For this review, take the finished solid that the model builds, in its own axes (mm). Coordinates: 2 decimals unless noted, no trailing zeros. Loops run counter-clockwise (first coordinate to the right, second up) from the corner with the lowest first, then second, coordinate; pieces in that order, holes last. Notation, with made-up numbers: (-10.5, 76) -> (38.5, 76) arc R28 cw to (38.5, 114) -> close; hole circle Ø9 at (-27.75, 15). An arc over 180 degrees is marked (long way). Use a Markdown table: item, result.
from build123d import *

# Parameters (mm, degrees)
CROQUIS1_W              = 580
CROQUIS1_H              = 80
CROQUIS1_R              = 12.6
SALIENTE_EXTRUIR1_DEPTH = 16


with BuildPart() as part:
    # Croquis1 → Saliente-Extruir1 (new body)
    with BuildSketch(Plane.XY):
        Rectangle(CROQUIS1_W, CROQUIS1_H)
        with Locations((-240, -20)):
            Circle(CROQUIS1_R, mode=Mode.SUBTRACT)
        with Locations((-120, -20)):
            Circle(CROQUIS1_R, mode=Mode.SUBTRACT)
        with Locations((0, -20)):
            Circle(CROQUIS1_R, mode=Mode.SUBTRACT)
        with Locations((120, -20)):
            Circle(CROQUIS1_R, mode=Mode.SUBTRACT)
        with Locations((240, -20)):
            Circle(CROQUIS1_R, mode=Mode.SUBTRACT)
    extrude(amount=-SALIENTE_EXTRUIR1_DEPTH)


solid = part.part
(1) Mouldability with a two-part tool opening along Y and no side actions: class faces 1 (the face through (-4, 40, -8)), 2 (the face through (227.412, -19.446, -7.888)), 3 (the face through (-4, 1, 0)) as pulls with the +Y half, pulls with the -Y half, needs draft (parallel to the pull), parting line crosses it, or undercut.
Found:
| item | result |
|---|---|
| face 1 | pulls with the +Y half |
| face 2 | undercut |
| face 3 | needs draft |
(2) For line 1 along X through (y, z) = (-18.5, -10.5); line 2 along Y through (x, z) = (-120, -6.75); line 3 along X through (y, z) = (-25.5, -10.75), list the stretches that pass through material, from the lowest coordinate up.
Found:
| item | result |
|---|---|
| line 1 | x = -290 to -252.51, -227.49 to -132.51, -107.49 to -12.51, 12.51 to 107.49, 132.51 to 227.49, 252.51 to 290 |
| line 2 | y = -40 to -32.6, -7.4 to 40 |
| line 3 | x = -290 to -251.34, -228.66 to -131.34, -108.66 to -11.34, 11.34 to 108.66, 131.34 to 228.66, 251.34 to 290 |
(3) Take a section at A-A on z = -4.5. Write out the cut boundary in (x, y), plus the area to 3 significant figures.
Found:
| item | result |
|---|---|
| outline | (-290, -40) -> (290, -40) -> (290, 40) -> (-290, 40) -> close; hole circle Ø25.2 at (-240, -20); hole circle Ø25.2 at (-120, -20); hole circle Ø25.2 at (0, -20); hole circle Ø25.2 at (120, -20); hole circle Ø25.2 at (240, -20) |
| area | 43,900 mm^2 |
(4) Take a section at C-C on y = -20. Write out the cut boundary in (x, z).
Found:
| item | result |
|---|---|
| outline | (-290, -16) -> (-252.6, -16) -> (-252.6, 0) -> (-290, 0) -> close; (-227.4, -16) -> (-132.6, -16) -> (-132.6, 0) -> (-227.4, 0) -> close; (-107.4, -16) -> (-12.6, -16) -> (-12.6, 0) -> (-107.4, 0) -> close; (12.6, -16) -> (107.4, -16) -> (107.4, 0) -> (12.6, 0) -> close; (132.6, -16) -> (227.4, -16) -> (227.4, 0) -> (132.6, 0) -> close; (252.6, -16) -> (290, -16) -> (290, 0) -> (252.6, 0) -> close |
(5) Take a section at B-B on x = 0. Write out the cut boundary in (y, z), plus the area to 3 significant figures.
Found:
| item | result |
|---|---|
| outline | (-40, -16) -> (-32.6, -16) -> (-32.6, 0) -> (-40, 0) -> close; (-7.4, -16) -> (40, -16) -> (40, 0) -> (-7.4, 0) -> close |
| area | 877 mm^2 |
